Geometry: see drawing. Coordinates: mm, zero at the bounding-box minimum. A direction names the side the tool comes from. Coordinates: 2 decimals unless noted, no trailing zeros. Loops run counter-clockwise (first coordinate to the right, second up) from the corner with the lowest first, then second, coordinate; pieces in that order, holes last. Notation, with made-up numbers: (-30.75, -34) - (-18.75, -34) arc R30 cw to (-18.75, 0) - close; hole circle Ø1 at (-28.5, 51). An arc over 180 degrees is marked (long way). Use one line per item in the form item = value.
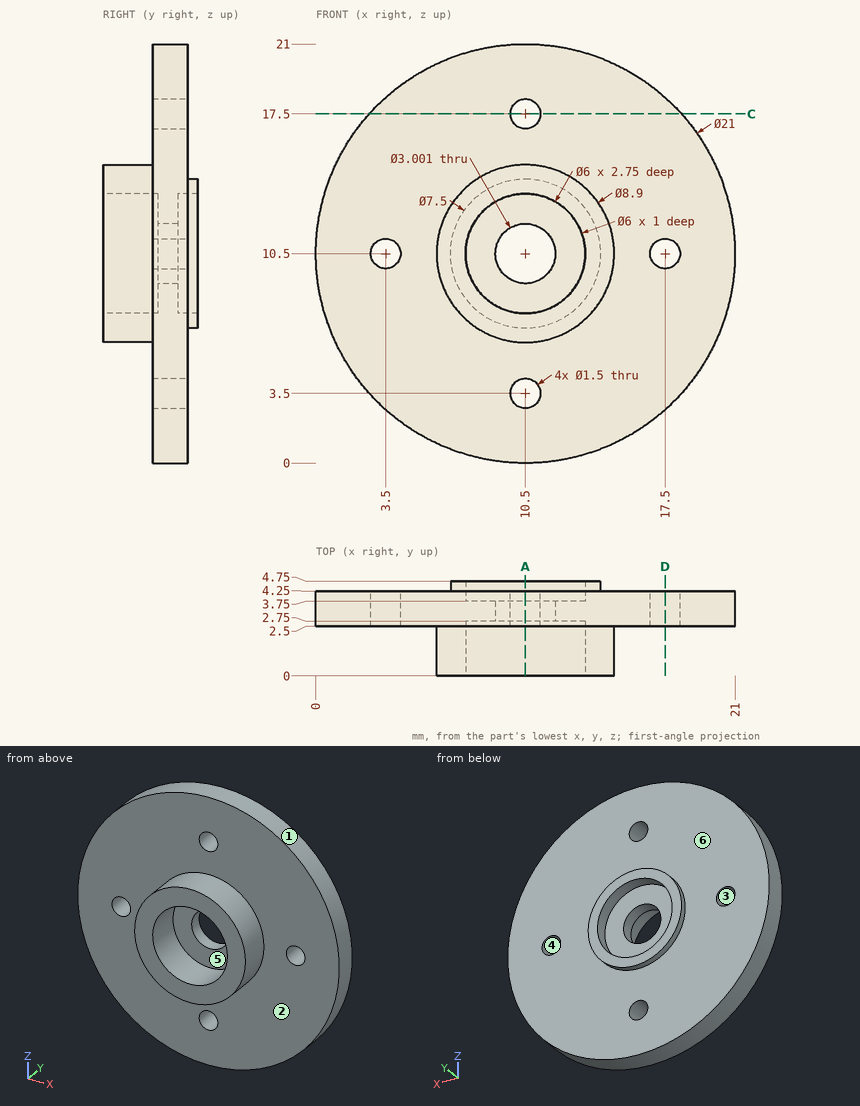
Q1. First-contact query: P1, Ø1.2, axis at x = 3.5, z = 10.5, coming from the -Y side (3 decimals); P2, Ø1.8, axis at x = 12, z = 11, coming from the -Y side; P3, Ø1.5, axis at x = 8.5, y = 2.5, coming from the +Z side; P4, Ø1, axis at x = 14, z = 6.5, coming from the +Y side. Flat tips, straight axial feed; report the tip coordinate or a pass-through.
Check values:
P1 = through
P2 = 2.75
P3 = 20.93
P4 = 4.25
Q2. Ray query, line 1 along X through (y, z) = (3, 10.5); line 2 along Y through (x, z) = (17.25, 6); line 3 along X through (y, z) = (4.3, 10.5). Return the intervals inside material, ascending. Write a range as [from, to].
Check values:
line_1 = [0, 2.75], [4.25, 9], [12, 16.75], [18.25, 21]
line_2 = [2.5, 4.25]
line_3 = [6.75, 7.5], [13.5, 14.25]
Q3. Cut plane C-C, the plane z = 17.5. Return loops of the section in (x, y).
Check values:
outline = (2.67, 2.5) - (9.75, 2.5) - (9.75, 4.25) - (2.67, 4.25) - close; (11.25, 2.5) - (18.33, 2.5) - (18.33, 4.25) - (11.25, 4.25) - close
Q4. Pull-direction query (Z, two-part tool) for the marked faces 1, 2 and 3; classes: pulls with the +Z half, pulls with the -Z half, needs draft (parallel to the pull), parting line crosses it, or undercut.
Check values:
face_1 = parting line crosses it
face_2 = needs draft
face_3 = undercut
Q5. Cut plane D-D, the plane x = 17.5. Return loops of the section in (y, z), then the cut area to 3 significant figures.
Check values:
outline = (2.5, 2.67) - (4.25, 2.67) - (4.25, 9.75) - (2.5, 9.75) - close; (2.5, 11.25) - (4.25, 11.25) - (4.25, 18.33) - (2.5, 18.33) - close
area = 24.8 mm²
Q6. Cut plane A-A, the plane x = 10.5. Give the number of separate pieces and of enclosed holes in the cut face, then the cut area to 3 significant figures.
Check values:
separate_pieces = 4
enclosed_holes = 0
area = 32.0 mm²
Q7. Set-up query: the marked faces 4, 5 and 6. Return all of +Z, -Z, +X, -X, +Y, -Y with unobstructed straight access to the full face (end or side cutting, diameter ignored); none if empty.
Check values:
face_4 = +Y, -Y
face_5 = -Y
face_6 = +Y
